```python
from build123d import *

# Parameters (mm, degrees)
SKETCH1_R                = 40
SKETCH1_R_2              = 5
BOSS_EXTRUDE1_DEPTH      = 5
SKETCH2_R                = 14.954923049
SKETCH2_R_2              = 5
BOSS_EXTRUDE2_DEPTH      = 30
SKETCH3_W                = 25
SKETCH3_H                = 35
BOSS_EXTRUDE3_DEPTH      = 65
BOSS_EXTRUDE4_DEPTH      = 12.5
BOSS_EXTRUDE4_DEPTH_BACK = 37.5
SKETCH4_R                = 15
SKETCH9_R                = 5
CUT_EXTRUDE5_DEPTH       = 111.566721937
SHELL14_START            = 2
SHELL14_OUTLINE_R        = 5
SHELL14_DEPTH            = 91
SHELL14_START_2          = 32
SHELL14_2_DEPTH          = 61
SHELL14_3_OUTLINE_R      = 38
SHELL14_3_DEPTH          = 1
SHELL14_START_3          = 3
SHELL14_4_DEPTH          = 30
SHELL14_START_4          = -23
SHELL14_5_OUTLINE_R      = 13
SHELL14_5_DEPTH          = 46
SKETCH11_R               = 1
CUT_EXTRUDE6_DEPTH       = 5
SKETCH10_R               = 5
CUT_EXTRUDE7_DEPTH       = 122.86057607
SKETCH12_W               = 25
SKETCH12_H               = 35
CUT_EXTRUDE8_DEPTH       = 2
SKETCH16_W               = 32.02314812
SKETCH16_H               = 50.956542264
CUT_EXTRUDE9_DEPTH       = 13


with BuildPart() as part:
    # Sketch1 → Boss-Extrude1 (new body)
    with BuildSketch(Plane(origin=(0, 0, 0), x_dir=(0, 0, -1), z_dir=(1, 0, 0))):
        Circle(SKETCH1_R)
        Circle(SKETCH1_R_2, mode=Mode.SUBTRACT)
    extrude(amount=BOSS_EXTRUDE1_DEPTH)

    # Sketch2 → Boss-Extrude2 (add)
    with BuildSketch(Plane(origin=(5, 0, 0), x_dir=(0, 0, -1), z_dir=(1, 0, 0))):
        Circle(SKETCH2_R)
        Circle(SKETCH2_R_2, mode=Mode.SUBTRACT)
    extrude(amount=BOSS_EXTRUDE2_DEPTH)

    # Sketch3 → Boss-Extrude3 (add)
    with BuildSketch(Plane(origin=(30, 0, 0), x_dir=(0, 0, -1), z_dir=(1, 0, 0))):
        Rectangle(SKETCH3_W, SKETCH3_H)
    extrude(amount=BOSS_EXTRUDE3_DEPTH)

    # Sketch4 → Boss-Extrude4 (add, two sides: drawn at the far end of the back side and taken through both)
    with BuildSketch(Plane(origin=(0, 0, -12.5), x_dir=(-1, 0, 0), z_dir=(0, 0, -1)).offset(-BOSS_EXTRUDE4_DEPTH_BACK)):
        with Locations((-65, 0)):
            Circle(SKETCH4_R)
    extrude(amount=BOSS_EXTRUDE4_DEPTH + BOSS_EXTRUDE4_DEPTH_BACK)

    # Sketch9 → Cut-Extrude5 (cut, through all)
    with BuildSketch(Plane.ZY):
        Circle(SKETCH9_R)
    extrude(amount=-CUT_EXTRUDE5_DEPTH, mode=Mode.SUBTRACT)

    # Shell14: read off the stored shape, not the designer's step
    # Shell14 outline → Shell14 (cut)
    with BuildSketch(Plane.YZ.offset(SHELL14_START)):
        with BuildLine():
            ThreePointArc((7.588150711, -10.5), (12.954923049, 0), (7.588150711, 10.5))
            Line((7.588150711, 10.5), (-7.588150711, 10.5))
            ThreePointArc((-7.588150711, 10.5), (-12.954923049, 0), (-7.588150711, -10.5))
            Line((-7.588150711, -10.5), (7.588150711, -10.5))
        make_face()
        Circle(SHELL14_OUTLINE_R, mode=Mode.SUBTRACT)
    extrude(amount=SHELL14_DEPTH, mode=Mode.SUBTRACT)

    # Shell14 2 outline → Shell14 2 (cut)
    with BuildSketch(Plane.YZ.offset(SHELL14_START_2)):
        with BuildLine():
            ThreePointArc((7.588150711, 10.5), (12.954923049, 0), (7.588150711, -10.5))
            Line((7.588150711, -10.5), (15.5, -10.5))
            Line((15.5, -10.5), (15.5, 10.5))
            Line((15.5, 10.5), (7.588150711, 10.5))
        make_face()
        with BuildLine():
            ThreePointArc((-7.588150711, -10.5), (-12.954923049, 0), (-7.588150711, 10.5))
            Line((-7.588150711, 10.5), (-15.5, 10.5))
            Line((-15.5, 10.5), (-15.5, -10.5))
            Line((-15.5, -10.5), (-7.588150711, -10.5))
        make_face()
    extrude(amount=SHELL14_2_DEPTH, mode=Mode.SUBTRACT)

    # Shell14 3 outline → Shell14 3 (cut)
    with BuildSketch(Plane.YZ.offset(SHELL14_START)):
        Circle(SHELL14_3_OUTLINE_R)
        with BuildLine():
            ThreePointArc((7.588150711, 10.5), (12.954923049, 0), (7.588150711, -10.5))
            Line((7.588150711, -10.5), (-7.588150711, -10.5))
            ThreePointArc((-7.588150711, -10.5), (-12.954923049, 0), (-7.588150711, 10.5))
            Line((-7.588150711, 10.5), (7.588150711, 10.5))
        make_face(mode=Mode.SUBTRACT)
    extrude(amount=SHELL14_3_DEPTH, mode=Mode.SUBTRACT)

    # Shell14 4 outline → Shell14 4 (cut)
    with BuildSketch(Plane.YZ.offset(SHELL14_START_3)):
        with BuildLine():
            Line((-7.588150711, 10.5), (7.588150711, 10.5))
            ThreePointArc((7.588150711, 10.5), (0, 12.954923049), (-7.588150711, 10.5))
        make_face()
        with BuildLine():
            ThreePointArc((-7.588150711, -10.5), (0, -12.954923049), (7.588150711, -10.5))
            Line((7.588150711, -10.5), (-7.588150711, -10.5))
        make_face()
    extrude(amount=SHELL14_4_DEPTH, mode=Mode.SUBTRACT)

    # Shell14 5 outline → Shell14 5 (cut)
    with BuildSketch(Plane.XY.offset(SHELL14_START_4)):
        with Locations((65, 0)):
            Circle(SHELL14_5_OUTLINE_R)
    extrude(amount=SHELL14_5_DEPTH, mode=Mode.SUBTRACT)

    # Sketch11 → Cut-Extrude6 (cut)
    with BuildSketch(Plane.ZY):
        with Locations((0, 7.5)):
            Circle(SKETCH11_R)
        with Locations((7.5, 0)):
            Circle(SKETCH11_R)
        with Locations((0, -7.5)):
            Circle(SKETCH11_R)
        with Locations((-7.5, 0)):
            Circle(SKETCH11_R)
    extrude(amount=-CUT_EXTRUDE6_DEPTH, mode=Mode.SUBTRACT)

    # Sketch10 → Cut-Extrude7 (cut, through all)
    with BuildSketch(Plane.XY.offset(25)):
        with Locations((65, 0)):
            Circle(SKETCH10_R)
    extrude(amount=-CUT_EXTRUDE7_DEPTH, mode=Mode.SUBTRACT)

    # Sketch12 → Cut-Extrude8 (cut)
    with BuildSketch(Plane(origin=(95, 0, 0), x_dir=(0, 0, -1), z_dir=(1, 0, 0))):
        Rectangle(SKETCH12_W, SKETCH12_H)
    extrude(amount=-CUT_EXTRUDE8_DEPTH, mode=Mode.SUBTRACT)

    # Sketch16 → Cut-Extrude9 (cut)
    with BuildSketch(Plane(origin=(93, 0, 0), x_dir=(0, 0, -1), z_dir=(1, 0, 0))):
        with Locations((0.70123682, -2.512765272)):
            Rectangle(SKETCH16_W, SKETCH16_H)
    extrude(amount=-CUT_EXTRUDE9_DEPTH, mode=Mode.SUBTRACT)


solid = part.part
```
Design review of the part built by this model. Coordinates are the model's own, in mm. A direction names the side the tool comes from. Round coordinates to 2 decimals unless told otherwise and drop trailing zeros. Write each loop counter-clockwise with the first axis right and the second up, starting at its lowest first coordinate (ties: lowest second). Pieces come first, ordered by that corner, then holes. Notation, with made-up numbers: (-2.5, 71) -> (31.5, 71) arc R23 cw to (31.5, 83) -> close; hole circle Ø1 at (25.25, -8.75). An arc over 180 degrees is marked (long way). Write item = value, one per line. Start each with the question number.
1) Tool access review of faces 4 (the face through (79.985, 0.66, 18.838)), 5 (the face through (3, 16, 1)), 6 (the face through (30, 16, 0)), 7 (the face through (79.985, 0.66, -18.662)), 8 (the face through (32, 13.2, 0.1)): name each direction out of +Z, -Z, +X, -X, +Y, -Y from which nothing blocks a thin tool from reaching the whole face with its end or side.
2) Take a section at A-A, the plane z = 19. State the section outline as (x, y) points, plus the area to 3 significant figures.
3) Wall thickness on probe 1 along X at (y, z) = (14, -12); probe 2 along Y at (x, z) = (65, -24.6); probe 3 along X at (y, z) = (-1, -32): over which ranges is each line inside the solid? List them lowest first. Write a range as from..to.
4) Clearance check with flat-ended pins moving along their axes: pin 1 (1 mm diameter, centred on x = 52, z = -0.5, fed in from -Y); pin 2 (20 mm diameter, centred on x = 64.5, z = -4, fed in from +Y); pin 3 (9 mm diameter, centred on x = 58, y = 7, fed in from +Z). State where each tip first meets the part, or that it passes through.
5) Take a section at C-C, the plane y = -24.5. State the section outline as (x, z) points.
6) Mouldability with a two-part tool opening along Z and no side actions: class faces 1 (the face through (69.619, -1.915, 24.014)), 2 (the face through (56, -15.5, 0)), 3 (the face through (69, 4, 25)) as +Z half, -Z half, draft (parallel to the pull), parting line (faces both ways), or undercut.
7) Take a section at D-D, the plane z = 27. State the section outline as (x, y) points, plus the area to 3 significant figures.
8) Take a section at B-B, the plane x = 15. State the section outline as (y, z) points, plus the area to 3 significant figures.
Results list:
q1.face_4 = +Z
q1.face_5 = none
q1.face_6 = +Y
q1.face_7 = -Z
q1.face_8 = +X
q2.outline = (0, -35.2) -> (5, -35.2) -> (5, 35.2) -> (0, 35.2) -> close; circle Ø30 at (65, 0); hole (2, -32.91) -> (3, -32.91) -> (3, 32.91) -> (2, 32.91) -> close; hole circle Ø26 at (65, 0)
q2.area = 462 mm²
q3.probe_1 = 0..2, 3..5, 30..80
q3.probe_2 = -15..-5, 5..15
q3.probe_3 = 0..2, 3..5
q4.pin_1 = -17.5
q4.pin_2 = 17.5
q4.pin_3 = 25
q5.outline = (0, -31.62) -> (5, -31.62) -> (5, 31.62) -> (0, 31.62) -> close; hole (2, -29.05) -> (3, -29.05) -> (3, 29.05) -> (2, 29.05) -> close
q6.face_1 = draft
q6.face_2 = undercut
q6.face_3 = +Z half
q7.outline = (0, -29.51) -> (5, -29.51) -> (5, 29.51) -> (0, 29.51) -> close; hole (2, -26.74) -> (3, -26.74) -> (3, 26.74) -> (2, 26.74) -> close
q7.area = 242 mm²
q8.outline = circle Ø29.91 at (0, 0); hole circle Ø25.91 at (0, 0)
q8.area = 175 mm²
